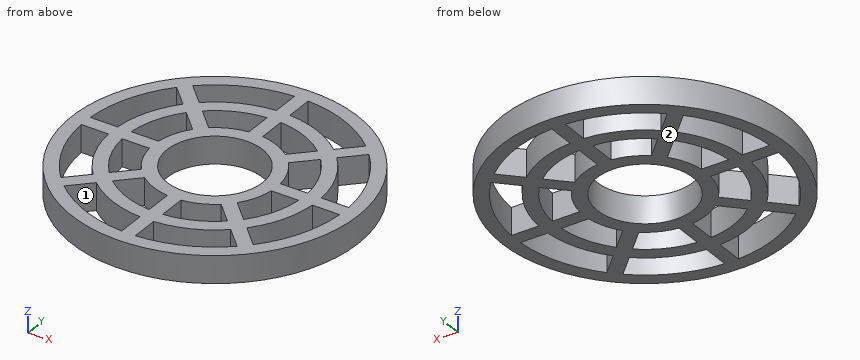
```python
from build123d import *

# Parameters (mm, degrees)
F0_R     = 13.335
F0_R_2   = 4.445
F1_DEPTH = 2.54
F3_DEPTH = 2.541


with BuildPart() as f1:
    # F0 (on Top) → F1 (new body)
    with BuildSketch(Plane.XY):
        Circle(F0_R)
        Circle(F0_R_2, mode=Mode.SUBTRACT)
    extrude(amount=F1_DEPTH)

    # F2 (on face) → F3 (cut, through all)
    with BuildSketch(Plane.XY.offset(2.54)):
        with BuildLine():
            ThreePointArc((-0.635, -5.679613), (-2.187036, -5.279972), (-3.56708, -4.465105))
            Line((-3.56708, -4.465105), (-5.368491, -6.266516))
            ThreePointArc((-5.368491, -6.266516), (-3.157774, -7.623541), (-0.635, -8.227192))
            Line((-0.635, -8.227192), (-0.635, -5.679613))
        make_face()
        with BuildLine():
            Line((-6.26883, -7.166855), (-8.070406, -8.968432))
            ThreePointArc((-8.070406, -8.968432), (-4.617076, -11.146607), (-0.635, -12.048278))
            Line((-0.635, -12.048278), (-0.635, -9.500464))
            ThreePointArc((-0.635, -9.500464), (-3.643782, -8.796868), (-6.26883, -7.166855))
        make_face()
        with BuildLine():
            Line((0.635, -5.679613), (0.635, -8.227192))
            ThreePointArc((0.635, -8.227192), (3.157774, -7.623541), (5.368491, -6.266516))
            Line((5.368491, -6.266516), (3.56708, -4.465105))
            ThreePointArc((3.56708, -4.465105), (2.187036, -5.279972), (0.635, -5.679613))
        make_face()
        with BuildLine():
            Line((0.635, -9.500464), (0.635, -12.048278))
            ThreePointArc((0.635, -12.048278), (4.617076, -11.146607), (8.070406, -8.968432))
            Line((8.070406, -8.968432), (6.26883, -7.166855))
            ThreePointArc((6.26883, -7.166855), (3.643782, -8.796868), (0.635, -9.500464))
        make_face()
        with BuildLine():
            Line((4.465105, -3.56708), (6.266516, -5.368491))
            ThreePointArc((6.266516, -5.368491), (7.623541, -3.157774), (8.227192, -0.635))
            Line((8.227192, -0.635), (5.679613, -0.635))
            ThreePointArc((5.679613, -0.635), (5.279972, -2.187036), (4.465105, -3.56708))
        make_face()
        with BuildLine():
            Line((7.166855, -6.26883), (8.968432, -8.070406))
            ThreePointArc((8.968432, -8.070406), (11.146607, -4.617076), (12.048278, -0.635))
            Line((12.048278, -0.635), (9.500464, -0.635))
            ThreePointArc((9.500464, -0.635), (8.796868, -3.643782), (7.166855, -6.26883))
        make_face()
        with BuildLine():
            Line((5.679613, 0.635), (8.227192, 0.635))
            ThreePointArc((8.227192, 0.635), (7.623541, 3.157774), (6.266516, 5.368491))
            Line((6.266516, 5.368491), (4.465105, 3.56708))
            ThreePointArc((4.465105, 3.56708), (5.279972, 2.187036), (5.679613, 0.635))
        make_face()
        with BuildLine():
            Line((9.500464, 0.635), (12.048278, 0.635))
            ThreePointArc((12.048278, 0.635), (11.146607, 4.617076), (8.968432, 8.070406))
            Line((8.968432, 8.070406), (7.166855, 6.26883))
            ThreePointArc((7.166855, 6.26883), (8.796868, 3.643782), (9.500464, 0.635))
        make_face()
        with BuildLine():
            Line((3.56708, 4.465105), (5.368491, 6.266516))
            ThreePointArc((5.368491, 6.266516), (3.157774, 7.623541), (0.635, 8.227192))
            Line((0.635, 8.227192), (0.635, 5.679613))
            ThreePointArc((0.635, 5.679613), (2.187036, 5.279972), (3.56708, 4.465105))
        make_face()
        with BuildLine():
            Line((6.26883, 7.166855), (8.070406, 8.968432))
            ThreePointArc((8.070406, 8.968432), (4.617076, 11.146607), (0.635, 12.048278))
            Line((0.635, 12.048278), (0.635, 9.500464))
            ThreePointArc((0.635, 9.500464), (3.643782, 8.796868), (6.26883, 7.166855))
        make_face()
        with BuildLine():
            Line((-0.635, 5.679613), (-0.635, 8.227192))
            ThreePointArc((-0.635, 8.227192), (-3.157774, 7.623541), (-5.368491, 6.266516))
            Line((-5.368491, 6.266516), (-3.56708, 4.465105))
            ThreePointArc((-3.56708, 4.465105), (-2.187036, 5.279972), (-0.635, 5.679613))
        make_face()
        with BuildLine():
            Line((-0.635, 9.500464), (-0.635, 12.048278))
            ThreePointArc((-0.635, 12.048278), (-4.617076, 11.146607), (-8.070406, 8.968432))
            Line((-8.070406, 8.968432), (-6.26883, 7.166855))
            ThreePointArc((-6.26883, 7.166855), (-3.643782, 8.796868), (-0.635, 9.500464))
        make_face()
        with BuildLine():
            Line((-4.465105, 3.56708), (-6.266516, 5.368491))
            ThreePointArc((-6.266516, 5.368491), (-7.623541, 3.157774), (-8.227192, 0.635))
            Line((-8.227192, 0.635), (-5.679613, 0.635))
            ThreePointArc((-5.679613, 0.635), (-5.279972, 2.187036), (-4.465105, 3.56708))
        make_face()
        with BuildLine():
            Line((-7.166855, 6.26883), (-8.968432, 8.070406))
            ThreePointArc((-8.968432, 8.070406), (-11.146607, 4.617076), (-12.048278, 0.635))
            Line((-12.048278, 0.635), (-9.500464, 0.635))
            ThreePointArc((-9.500464, 0.635), (-8.796868, 3.643782), (-7.166855, 6.26883))
        make_face()
        with BuildLine():
            Line((-5.679613, -0.635), (-8.227192, -0.635))
            ThreePointArc((-8.227192, -0.635), (-7.623541, -3.157774), (-6.266516, -5.368491))
            Line((-6.266516, -5.368491), (-4.465105, -3.56708))
            ThreePointArc((-4.465105, -3.56708), (-5.279972, -2.187036), (-5.679613, -0.635))
        make_face()
        with BuildLine():
            Line((-9.500464, -0.635), (-12.048278, -0.635))
            ThreePointArc((-12.048278, -0.635), (-11.146607, -4.617076), (-8.968432, -8.070406))
            Line((-8.968432, -8.070406), (-7.166855, -6.26883))
            ThreePointArc((-7.166855, -6.26883), (-8.796868, -3.643782), (-9.500464, -0.635))
        make_face()
    extrude(amount=-F3_DEPTH, mode=Mode.SUBTRACT)


solid = f1.part
```
The listing builds one solid part. Answer for the finished solid, in the listing's coordinates (mm). Face numbers are marked on the shaded views. Give positions to 0.01 mm unless a question says otherwise; leave off trailing zeros. Order: outer loops, then holes, each group sorted by start corner. A loop starts at its lowest first (then second) coordinate and runs counter-clockwise, first axis right, second up. Notation, with made-up numbers: (-33.5, -9) - (14.5, -9) arc R22 ccw to (14.5, 28) - close; hole circle Ø11 at (-5.5, 40.25). An arc over 180 degrees is marked (long way). Answer in a Markdown table with one row per item. Add a question column.
Q1. The part is cut by section C-C (x = -7.5). Determine the outline of the cut face in (y, z) (3 decimals), then the cut area to 3 significant figures.
Q2. Find the intervals of material crossed by line 1 along Y through (x, z) = (0, 0.75) (3 decimals); line 2 along Y through (x, z) = (-6.5, 0.85) (3 decimals); line 3 along X through (y, z) = (-1.25, 0.6), in increasing order. Write a range as [from, to].
Q3. For a pull along Y with two mould halves and no side action, classify the marked faces 1 and 2 as released by +Y, released by -Y, zero draft, split by the parting line, or undercut.
Q4. The part is cut by section A-A (y = 0). Determine the outline of the cut face in (x, z) (3 decimals), then the cut area to 3 significant figures.
Q5. The part is cut by section D-D (x = 6.75). Determine the outline of the cut face in (y, z) (3 decimals), then the cut area to 3 significant figures.
Q6. Given P1, Ø0.8, axis at x = -10.5, z = 2, coming from the +Y side; P2, Ø1.3, axis at x = 11.5, z = 1.5, coming from the +Y side; P3, Ø1.5, axis at x = 1.5, z = 1, coming from the +Y side, each flat-ended and moving along its own axis, determine where each tip first touches the part or whether it passes through.
Determined:
| question | item | result |
|---|---|---|
| 1 | outline | (-11.026, 0) - (-9.451, 0) - (-9.451, 2.54) - (-11.026, 2.54) - close; (-8.398, 0) - (-6.602, 0) - (-6.602, 2.54) - (-8.398, 2.54) - close; (-5.866, 0) - (-3.441, 0) - (-3.441, 2.54) - (-5.866, 2.54) - close; (-0.635, 0) - (0.635, 0) - (0.635, 2.54) - (-0.635, 2.54) - close; (3.441, 0) - (5.866, 0) - (5.866, 2.54) - (3.441, 2.54) - close; (6.602, 0) - (8.398, 0) - (8.398, 2.54) - (6.602, 2.54) - close; (9.451, 0) - (11.026, 0) - (11.026, 2.54) - (9.451, 2.54) - close |
| 1 | area | 32.7 mm² |
| 2 | line 1 | y = [-13.335, -4.445], [4.445, 13.335] |
| 2 | line 2 | y = [-11.644, -10.164], [-7.398, -5.083], [-0.635, 0.635], [5.083, 7.398], [10.164, 11.644] |
| 2 | line 3 | x = [-13.28, -12], [-9.44, -8.16], [-5.58, -4.27], [4.27, 5.58], [8.16, 9.44], [12, 13.28] |
| 3 | face 1 | undercut |
| 3 | face 2 | zero draft |
| 4 | outline | (-13.335, 0) - (-4.445, 0) - (-4.445, 2.54) - (-13.335, 2.54) - close; (4.445, 0) - (13.335, 0) - (13.335, 2.54) - (4.445, 2.54) - close |
| 4 | area | 45.2 mm² |
| 5 | outline | (-11.5, 0) - (-10, 0) - (-10, 2.54) - (-11.5, 2.54) - close; (-7.648, 0) - (-4.746, 0) - (-4.746, 2.54) - (-7.648, 2.54) - close; (-0.635, 0) - (0.635, 0) - (0.635, 2.54) - (-0.635, 2.54) - close; (4.746, 0) - (7.648, 0) - (7.648, 2.54) - (4.746, 2.54) - close; (10, 0) - (11.5, 0) - (11.5, 2.54) - (10, 2.54) - close |
| 5 | area | 25.6 mm² |
| 6 | P1 | stops at y = 8.71 |
| 6 | P2 | stops at y = 7.75 |
| 6 | P3 | stops at y = 13.31 |
